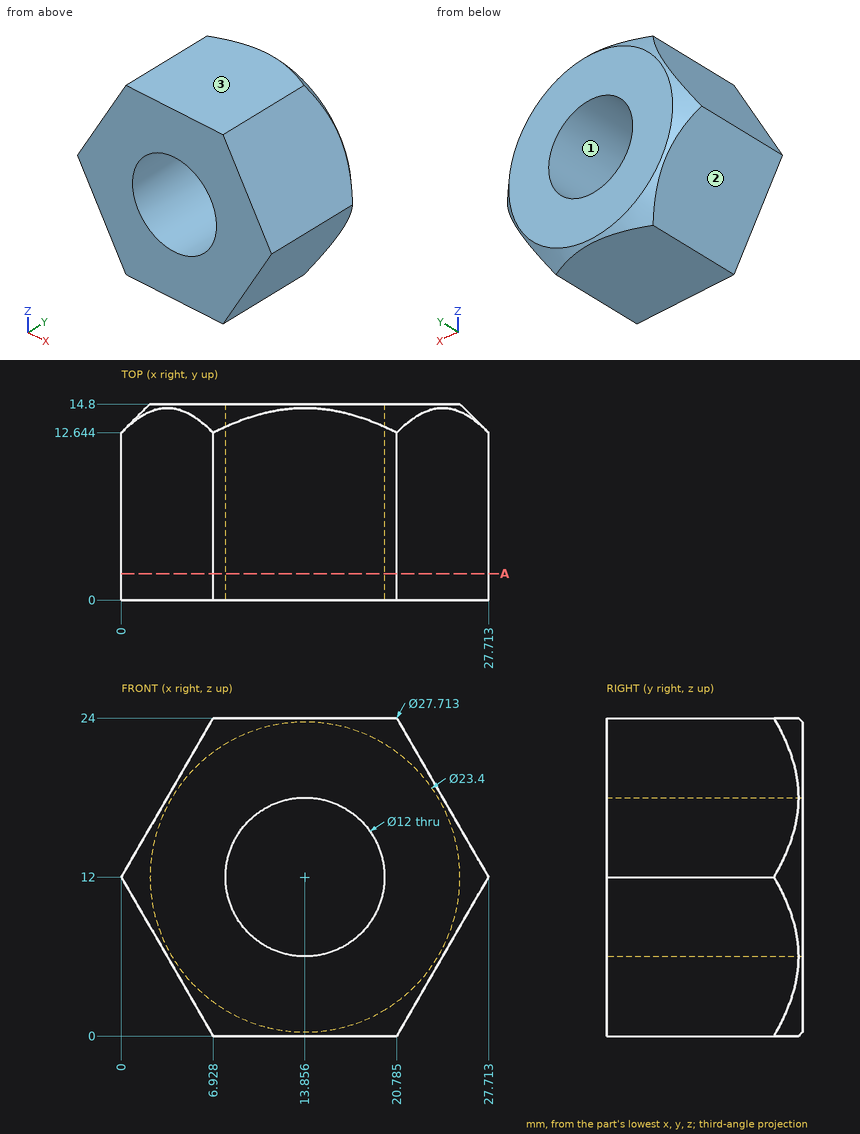
Study the drawing (mm; zero at the part's minimum x, y, z) and answer. Round coordinates to 2 decimals unless told otherwise and drop trailing zeros. Write each loop counter-clockwise with the first axis right and the second up, starting at its lowest first coordinate (ties: lowest second). Pieces come first, ordered by that corner, then holes. Notation, with made-up numbers: (71.5, -38) - (123.5, -38) arc R15 cw to (123.5, -18) - close; hole circle Ø8 at (87.25, 7). An arc over 180 degrees is marked (long way). Use CSV: the item, a comma, the result in double quotes.
Q1. This flat-tipped pin is pushed along its axis until it touches: pin 1 Ø11 at (x, z) = (13.86, 12) entering from -Y (1 decimal). Where does it stop, or does it pass through?
Values:
pin 1,"passes through"
Q2. Determine the mould class of the marked faces 1, 2 and 3 for opening direction X: +X half, -X half, draft (parallel to the pull), parting line (faces both ways), or undercut.
Values:
face 1,"undercut"
face 2,"-X half"
face 3,"draft"
Q3. Find section A-A, the plane y = 2. Write down the section's boundary in (x, z) (1 decimal).
Values:
outline,"(0, 12) - (6.9, 0) - (20.8, 0) - (27.7, 12) - (20.8, 24) - (6.9, 24) - close; hole circle Ø12 at (13.9, 12)"
Q4. Straight lines are drawn through the part: line 1 along Z through (x, y) = (11.75, 13); line 2 along X through (y, z) = (7, 16.25) (1 decimal); line 3 along Z through (x, y) = (18.75, 5.25). For each, find the intervals that lie inside material, in ascending order.
Values:
line 1,"z = 0 to 6.38, 17.62 to 24"
line 2,"x = 2.5 to 9.6, 18.1 to 25.3"
line 3,"z = 0 to 8.53, 15.47 to 24"
